from build123d import *

# Parameters (mm, degrees)
F0_R     = 4.975
F1_DEPTH = 3


with BuildPart() as f1:
    # F0 (on Right) → F1 (new body)
    with BuildSketch(Plane.YZ):
        with BuildLine():
            ThreePointArc((-14, 26), (-17.535534, 24.535534), (-19, 21))
            Line((-19, 21), (-19, 17.3))
            Line((-19, 17.3), (-11, 17.3))
            Line((-11, 17.3), (-11, -21.65))
            Line((-11, -21.65), (-19, -21.65))
            Line((-19, -21.65), (-19, -26))
            Line((-19, -26), (9, -26))
            ThreePointArc((9, -26), (16.071068, -23.071068), (19, -16))
            Line((19, -16), (19, 16))
            ThreePointArc((19, 16), (16.071068, 23.071068), (9, 26))
            Line((9, 26), (-14, 26))
        make_face()
        with Locations((4, -19)):
            Circle(F0_R, mode=Mode.SUBTRACT)
        with Locations((4, 0)):
            Circle(F0_R, mode=Mode.SUBTRACT)
        with Locations((4, 19)):
            Circle(F0_R, mode=Mode.SUBTRACT)
    extrude(amount=F1_DEPTH)


solid = f1.part
Input: part model. Units: mm. Frame: model coordinates. A direction names the side the tool comes from. Coordinates: 2 decimals unless noted, no trailing zeros. Loops run counter-clockwise (first coordinate to the right, second up) from the corner with the lowest first, then second, coordinate; pieces in that order, holes last. Notation, with made-up numbers: (60, -26.5) - (111, -26.5) arc R30 ccw to (111, -4.5) - close; hole circle Ø1 at (-39, 88.25). An arc over 180 degrees is marked (long way). Answer in a Markdown table with one row per item. Add a question column.
Item 1: Mould query, pull axis Y, two halves, no side actions, for faces 1 (the flat face through (1, -11, -2)), 2 (the cylindrical face through (1.479, 3.352, 23.933)), 3 (the flat face through (3, 0, 6)). Classes: released by +Y, released by -Y, zero draft, split by the parting line, or undercut.
Item 2: Section query B-B on z = 0. Return the cut outline in (x, y) (3 decimals), then the cut area to 4 significant figures.
Item 3: Section query C-C on y = 4. Return the cut outline in (x, z) (3 decimals).
Item 4: Line query: line 1 along Z through (x, y) = (0.8, 4) (3 decimals); line 2 along Z through (x, y) = (0.3, 6); line 3 along Y through (x, z) = (2.6, 13). Output: solid intervals per line, ascending. Write a range as [from, to].
Item 5: Contact query for flat-ended pins moving along their axis: P1, Ø1, axis at x = 0.5, z = -13.5, coming from the -Y side; P2, Ø9, axis at y = 4, z = -19, coming from the +X side; P3, Ø8, axis at y = -3, z = -18, coming from the -X side. Output: stop coordinate, or through.
Item 6: Access query for faces 4 (the cylindrical face through (1.479, 3.352, -14.067)), 5 (the flat face through (1, -15, 17.3)). Directions: +Z, -Z, +X, -X, +Y, -Y. A direction counts if a zero-diameter tool reaches every point of the face in a straight line with its end or side. Return the directions, or none.
Item 7: Section query D-D on z = -6.5. Return the cut outline in (x, y).
Item 8: Section query A-A on x = 0.8. Return the cut outline in (y, z) (3 decimals).
Recorded:
| question | item | result |
|---|---|---|
| 1 | face 1 | released by -Y |
| 1 | face 2 | undercut |
| 1 | face 3 | zero draft |
| 2 | outline | (0, -11) - (3, -11) - (3, -0.975) - (0, -0.975) - close; (0, 8.975) - (3, 8.975) - (3, 19) - (0, 19) - close |
| 2 | area | 60.15 mm^2 |
| 3 | outline | (0, -26) - (3, -26) - (3, -23.975) - (0, -23.975) - close; (0, -14.025) - (3, -14.025) - (3, -4.975) - (0, -4.975) - close; (0, 4.975) - (3, 4.975) - (3, 14.025) - (0, 14.025) - close; (0, 23.975) - (3, 23.975) - (3, 26) - (0, 26) - close |
| 4 | line 1 | [-26, -23.975], [-14.025, -4.975], [4.975, 14.025], [23.975, 26] |
| 4 | line 2 | [-26, -23.56], [-14.44, -4.56], [4.56, 14.44], [23.56, 26] |
| 4 | line 3 | [-11, 19] |
| 5 | P1 | y = -11 |
| 5 | P2 | through |
| 5 | P3 | x = 0 |
| 6 | face 4 | +X, -X |
| 6 | face 5 | +X, -X, -Y |
| 7 | outline | (0, -11) - (3, -11) - (3, 19) - (0, 19) - close |
| 8 | outline | (-19, -26) - (9, -26) arc R10 ccw to (19, -16) - (19, 16) arc R10 ccw to (9, 26) - (-14, 26) arc R5 ccw to (-19, 21) - (-19, 17.3) - (-11, 17.3) - (-11, -21.65) - (-19, -21.65) - close; hole circle Ø9.95 at (4, -19); hole circle Ø9.95 at (4, 0); hole circle Ø9.95 at (4, 19) |
